Part model, mm, in its own coordinate system. Face numbers are marked on the shaded views. A direction names the side the tool comes from. Give positions to 0.01 mm unless a question says otherwise; leave off trailing zeros. Order: outer loops, then holes, each group sorted by start corner. A loop starts at its lowest first (then second) coordinate and runs counter-clockwise, first axis right, second up. Notation, with made-up numbers: M 56.25,-25 L 80.25,-25 A23 cw 80.25,-10 Z; hole C -37.5,-15 d10. An arc over 180 degrees is marked long. Write each question's results on one line, items separated by ' | '. Start each with the question number.
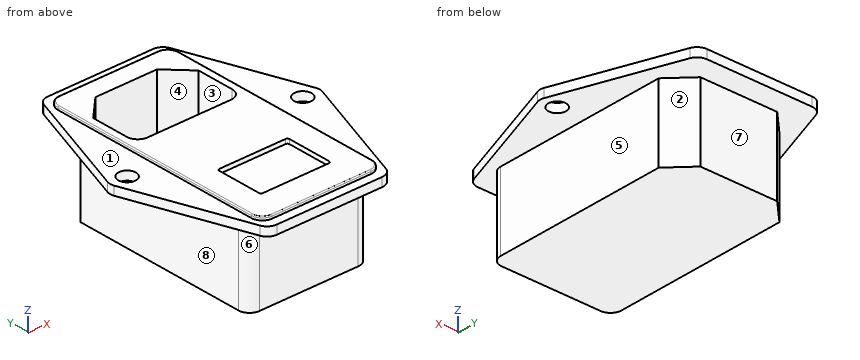
from build123d import *

# Parameters (mm, degrees)
SKETCH1_R           = 2
BOSS_EXTRUDE1_DEPTH = 2
BOSS_EXTRUDE2_DEPTH = 0.75
FILLET1_R           = 0.25
BOSS_EXTRUDE3_DEPTH = 17.5
CUT_EXTRUDE1_DEPTH  = 17.5
CUT_EXTRUDE2_DEPTH  = 1


with BuildPart() as part:
    # Sketch1 → Boss-Extrude1 (new body)
    with BuildSketch(Plane.XY):
        with BuildLine():
            Line((28.089158303, 56.333113093), (37.455537614, 29.833113093))
            ThreePointArc((37.455537614, 29.833113093), (37.598437155, 29), (37.455537614, 28.166886907))
            Line((37.455537614, 28.166886907), (28.089158303, 1.666886907))
            ThreePointArc((28.089158303, 1.666886907), (27.175528881, 0.458825983), (25.732057844, 0))
            Line((25.732057844, 0), (1.767942156, 0))
            ThreePointArc((1.767942156, 0), (0.324471119, 0.458825983), (-0.589158303, 1.666886907))
            Line((-0.589158303, 1.666886907), (-9.955537614, 28.166886907))
            ThreePointArc((-9.955537614, 28.166886907), (-10.098437155, 29), (-9.955537614, 29.833113093))
            Line((-9.955537614, 29.833113093), (-0.589158303, 56.333113093))
            ThreePointArc((-0.589158303, 56.333113093), (0.324471119, 57.541174017), (1.767942156, 58))
            Line((1.767942156, 58), (25.732057844, 58))
            ThreePointArc((25.732057844, 58), (27.175528881, 57.541174017), (28.089158303, 56.333113093))
        make_face()
        with Locations((-6.25, 29)):
            Circle(SKETCH1_R, mode=Mode.SUBTRACT)
        with Locations((33.75, 29)):
            Circle(SKETCH1_R, mode=Mode.SUBTRACT)
    extrude(amount=BOSS_EXTRUDE1_DEPTH)

    # Sketch2 → Boss-Extrude2 (add)
    with BuildSketch(Plane.XY.offset(2)):
        with BuildLine():
            Line((2.5, 2), (25, 2))
            ThreePointArc((25, 2), (26.767766953, 2.732233047), (27.5, 4.5))
            Line((27.5, 4.5), (27.5, 53.5))
            ThreePointArc((27.5, 53.5), (26.767766953, 55.267766953), (25, 56))
            Line((25, 56), (2.5, 56))
            ThreePointArc((2.5, 56), (0.732233047, 55.267766953), (0, 53.5))
            Line((0, 53.5), (0, 4.5))
            ThreePointArc((0, 4.5), (0.732233047, 2.732233047), (2.5, 2))
        make_face()
    extrude(amount=BOSS_EXTRUDE2_DEPTH)

    # Fillet1
    fillet1_edges = [part.edges().sort_by_distance(p)[0] for p in [
        (0.732233047, 2.732233047, 2.75),
        (13.75, 2, 2.75),
        (26.767766953, 2.732233047, 2.75),
        (27.5, 29, 2.75),
        (26.767766953, 55.267766953, 2.75),
        (13.75, 56, 2.75),
        (0.732233047, 55.267766953, 2.75),
        (0, 29, 2.75),
    ]]
    fillet(fillet1_edges, radius=FILLET1_R)

    # Sketch3 → Boss-Extrude3 (add)
    with BuildSketch(Plane(origin=(0, 0, 0), x_dir=(-1, 0, 0), z_dir=(0, 0, -1))):
        with BuildLine():
            Line((-27.5, 47.75), (-22.5, 52.75))
            Line((-22.5, 52.75), (-5, 52.75))
            Line((-5, 52.75), (0, 47.75))
            Line((0, 47.75), (0, 7.75))
            ThreePointArc((0, 7.75), (-0.732233047, 5.982233047), (-2.5, 5.25))
            Line((-2.5, 5.25), (-25, 5.25))
            ThreePointArc((-25, 5.25), (-26.767766953, 5.982233047), (-27.5, 7.75))
            Line((-27.5, 7.75), (-27.5, 47.75))
        make_face()
    extrude(amount=BOSS_EXTRUDE3_DEPTH)

    # Sketch4 → Cut-Extrude1 (cut)
    with BuildSketch(Plane.XY.offset(2.75)):
        with BuildLine():
            Line((1.75, 46.5), (6.75, 51.5))
            Line((6.75, 51.5), (20.75, 51.5))
            Line((20.75, 51.5), (25.75, 46.5))
            Line((25.75, 46.5), (25.75, 38))
            ThreePointArc((25.75, 38), (25.017766953, 36.232233047), (23.25, 35.5))
            Line((23.25, 35.5), (4.25, 35.5))
            ThreePointArc((4.25, 35.5), (2.482233047, 36.232233047), (1.75, 38))
            Line((1.75, 38), (1.75, 46.5))
        make_face()
    extrude(amount=-CUT_EXTRUDE1_DEPTH, mode=Mode.SUBTRACT)

    # Sketch5 → Cut-Extrude2 (cut)
    with BuildSketch(Plane.XY.offset(2.75)):
        with BuildLine():
            Line((6.25, 19.5), (21.25, 19.5))
            ThreePointArc((21.25, 19.5), (21.603553391, 19.353553391), (21.75, 19))
            Line((21.75, 19), (21.75, 9))
            ThreePointArc((21.75, 9), (21.603553391, 8.646446609), (21.25, 8.5))
            Line((21.25, 8.5), (6.25, 8.5))
            ThreePointArc((6.25, 8.5), (5.896446609, 8.646446609), (5.75, 9))
            Line((5.75, 9), (5.75, 19))
            ThreePointArc((5.75, 19), (5.896446609, 19.353553391), (6.25, 19.5))
        make_face()
    extrude(amount=-CUT_EXTRUDE2_DEPTH, mode=Mode.SUBTRACT)


solid = part.part
(1) Saw through at D-D on z = -6.5. Give the cut face in (x, y), plus the area to 3 significant figures.
(2) Drop flat-ended pins along their axis: P1, Ø6.5, axis at x = -6.25, y = 29, coming from the +Z side; P2, Ø2.5, axis at y = 42, z = -7, coming from the -X side; P3, Ø5, axis at x = 17, y = 39.5, coming from the +Z side. Give the stop position or say it passes through.
(3) Saw through at A-A on y = 29. Give the cut face in (x, z).
(4) Saw through at B-B on z = 1. Give the cut face in (x, y).
(5) Pull direction Y, two halves, no side cores. Call the marked faces 1, 2 and 3: +Y half, -Y half, draft (parallel to the pull), parting line (faces both ways), or undercut.
(6) Saw through at C-C on x = 33.75. Give the cut face in (y, z), plus the area to 3 significant figures.
(7) Tool access for the marked faces 4, 5, 6, 7 and 8: list every direction of +Z, -Z, +X, -X, +Y, -Y with a clear straight run to the whole face (end or side of a thin tool).
(8) Probe L1, parallel to X at y = 38, z = -11.75; L2, parallel to Y at x = 9, z = -11. List the from-to ranges inside material, lowest first.
Taken from the geometry:
1) outline: M 0,7.75 A2.5 ccw 2.5,5.25 L 25,5.25 A2.5 ccw 27.5,7.75 L 27.5,47.75 L 22.5,52.75 L 5,52.75 L 0,47.75 Z; hole M 1.75,38 A2.5 ccw 4.25,35.5 L 23.25,35.5 A2.5 ccw 25.75,38 L 25.75,46.5 L 20.75,51.5 L 6.75,51.5 L 1.75,46.5 Z | area: 922 mm²
2) P1: stops at z = 2 | P2: stops at x = 0 | P3: stops at z = -14.75
3) outline: M -10.1,0 L -8.25,0 L -8.25,2 L -10.1,2 Z; M -4.25,0 L 0,0 L 0,-17.5 L 27.5,-17.5 L 27.5,0 L 31.75,0 L 31.75,2 L 27.5,2 L 27.5,2.5 A0.25 ccw 27.25,2.75 L 0.25,2.75 A0.25 ccw 0,2.5 L 0,2 L -4.25,2 Z; M 35.75,0 L 37.6,0 L 37.6,2 L 35.75,2 Z
4) outline: M -9.96,28.17 L -0.59,1.67 A2.5 ccw 1.77,0 L 25.73,0 A2.5 ccw 28.09,1.67 L 37.46,28.17 A2.5 ccw 37.46,29.83 L 28.09,56.33 A2.5 ccw 25.73,58 L 1.77,58 A2.5 ccw -0.59,56.33 L -9.96,29.83 A2.5 ccw Z; hole C -6.25,29 d4; hole M 1.75,38 A2.5 ccw 4.25,35.5 L 23.25,35.5 A2.5 ccw 25.75,38 L 25.75,46.5 L 20.75,51.5 L 6.75,51.5 L 1.75,46.5 Z; hole C 33.75,29 d4
5) face 1: draft | face 2: +Y half | face 3: undercut
6) outline: M 17.68,0 L 27,0 L 27,2 L 17.68,2 Z; M 31,0 L 40.32,0 L 40.32,2 L 31,2 Z | area: 37.3 mm²
7) face 4: +Z | face 5: -Z, +X, +Y, -Y | face 6: -Z, -X, -Y | face 7: -Z, +X, -X, +Y | face 8: -Z, -X, +Y, -Y
8) L1: x = 0 to 1.75, 25.75 to 27.5 | L2: y = 5.25 to 35.5, 51.5 to 52.75
